Verification items for the finished model (mm, model axes). Round coordinates to 2 decimals unless told otherwise and drop trailing zeros. Loops run counter-clockwise (first coordinate to the right, second up) from the corner with the lowest first, then second, coordinate; pieces in that order, holes last. Notation, with made-up numbers: (29.5, 41.25) - (39.5, 41.25) arc R29 cw to (39.5, 78.25) - close; hole circle Ø6 at (52.5, -5). An arc over 180 degrees is marked (long way). Use a Markdown table: item, result. Add a question column.
```python
from build123d import *

# Parameters (mm, degrees)
CROQUIS1_W                       = 200
CROQUIS1_H                       = 180
CROQUIS1_R                       = 57
CROQUIS1_R_2                     = 4
SALIENTE_EXTRUIR1_DEPTH          = 4
CROQUIS2_R                       = 61
CROQUIS2_R_2                     = 57
SALIENTE_EXTRUIR2_DEPTH          = 76
CROQUIS3_W                       = 8
CROQUIS3_H                       = 23.163617774
CORTAR_EXTRUIR1_DEPTH            = 50
TALADRO_DE_MARGEN_PARA_M81_D     = 9
TALADRO_DE_MARGEN_PARA_M81_DEPTH = 4.999


with BuildPart() as part:
    # Croquis1 → Saliente-Extruir1 (new body)
    with BuildSketch(Plane(origin=(0, 0, 0), x_dir=(0, 0, -1), z_dir=(1, 0, 0))):
        Rectangle(CROQUIS1_W, CROQUIS1_H)
        Circle(CROQUIS1_R, mode=Mode.SUBTRACT)
        with Locations((-57, 57)):
            Circle(CROQUIS1_R_2, mode=Mode.SUBTRACT)
        with Locations(Location((57, 57, 0), (0, 0, 180))):
            Circle(CROQUIS1_R_2, mode=Mode.SUBTRACT)
        with Locations((57, -57)):
            Circle(CROQUIS1_R_2, mode=Mode.SUBTRACT)
        with Locations(Location((-57, -57, 0), (0, 0, 180))):
            Circle(CROQUIS1_R_2, mode=Mode.SUBTRACT)
    extrude(amount=SALIENTE_EXTRUIR1_DEPTH)

    # Croquis2 → Saliente-Extruir2 (add)
    with BuildSketch(Plane(origin=(4, 0, 0), x_dir=(0, 0, -1), z_dir=(1, 0, 0))):
        Circle(CROQUIS2_R)
        Circle(CROQUIS2_R_2, mode=Mode.SUBTRACT)
    extrude(amount=SALIENTE_EXTRUIR2_DEPTH)

    # Croquis3 → Cortar-Extruir1 (cut)
    with BuildSketch(Plane(origin=(80, 0, 0), x_dir=(0, 0, -1), z_dir=(1, 0, 0))):
        with Locations((0, 57)):
            Rectangle(CROQUIS3_W, CROQUIS3_H)
        with Locations((0, -57)):
            Rectangle(CROQUIS3_W, CROQUIS3_H)
    extrude(amount=-CORTAR_EXTRUIR1_DEPTH, mode=Mode.SUBTRACT)

    # Taladro de margen para M81
    with Locations(Plane(origin=(4, -7.41730184, -252.760845032), x_dir=(0, 0, -1), z_dir=(1, 0, 0))):
        with Locations((-342.760845032, 71.41730184), (-342.760845032, 26.41730184), (-162.760845032, 73.414694032), (-162.760845032, 28.414694032), (-195.760845032, -49.58269816), (-309.760845032, -49.58269816)):
            Hole(TALADRO_DE_MARGEN_PARA_M81_D / 2, depth=TALADRO_DE_MARGEN_PARA_M81_DEPTH)


solid = part.part
```
Q1. Go/stop test with flat-tipped pins: pin 1 Ø5.5 at (y, z) = (-57, -57) entering from -X; pin 2 Ø4.5 at (x, y) = (57, 58.5) entering from -Z; pin 3 Ø2 at (x, z) = (21.5, -41.5) entering from +Y; pin 4 Ø8 at (x, y) = (38.5, -50.5) entering from +Z. Record where each tip stops, or that it passes through.
Q2. Section check C-C on z = 90. Record the cut outline in (x, y).
Q3. Section check A-A on y = 0. Record the cut outline in (x, z).
Q4. Section check D-D on z = 15. Record the cut outline in (x, y), plus the area to 3 significant figures.
Q5. Thickness scan on line 1 along Y through (x, z) = (1, 90); line 2 along X through (y, z) = (-63.5, 23); line 3 along Z through (x, y) = (13, -42.5). Record the ranges inside material, lowest first.
Q6. Release check for a two-part mould opening along Z. For faces 1 (the face through (41.468, -37.118, 48.408)), 2 (the face through (4, 61.3, 1.4)), 3 (the face through (1.972, 22.794, 92.419)) record: +Z half, -Z half, draft (parallel to the pull), parting line (faces both ways), or undercut.
Q7. Section check B-B on x = 35. Record the cut outline in (y, z).
Determined:
| question | item | result |
|---|---|---|
| 1 | pin 1 | passes through |
| 1 | pin 2 | stops at z = -23.6 |
| 1 | pin 3 | stops at y = 45.62 |
| 1 | pin 4 | stops at z = 39.48 |
| 2 | outline | (0, -90) - (4, -90) - (4, 14.5) - (0, 14.5) - close; (0, 23.5) - (4, 23.5) - (4, 59.5) - (0, 59.5) - close; (0, 68.5) - (4, 68.5) - (4, 90) - (0, 90) - close |
| 3 | outline | (0, -100) - (4, -100) - (4, -61) - (80, -61) - (80, -57) - (0, -57) - close; (0, 57) - (80, 57) - (80, 61) - (4, 61) - (4, 100) - (0, 100) - close |
| 4 | outline | (0, -90) - (4, -90) - (4, -59.13) - (80, -59.13) - (80, -54.99) - (0, -54.99) - close; (0, 54.99) - (80, 54.99) - (80, 59.13) - (4, 59.13) - (4, 90) - (0, 90) - close |
| 4 | area | 909 mm² |
| 5 | line 1 | y = -90 to 14.5, 23.5 to 59.5, 68.5 to 90 |
| 5 | line 2 | x = 0 to 4 |
| 5 | line 3 | z = -43.76 to -37.98, 37.98 to 43.76 |
| 6 | face 1 | parting line |
| 6 | face 2 | draft |
| 6 | face 3 | undercut |
| 7 | outline | (-60.87, -4) arc R61 ccw to (60.87, -4) - (56.86, -4) arc R57 cw to (-56.86, -4) - close; (-60.87, 4) - (-56.86, 4) arc R57 cw to (56.86, 4) - (60.87, 4) arc R61 ccw to start |
